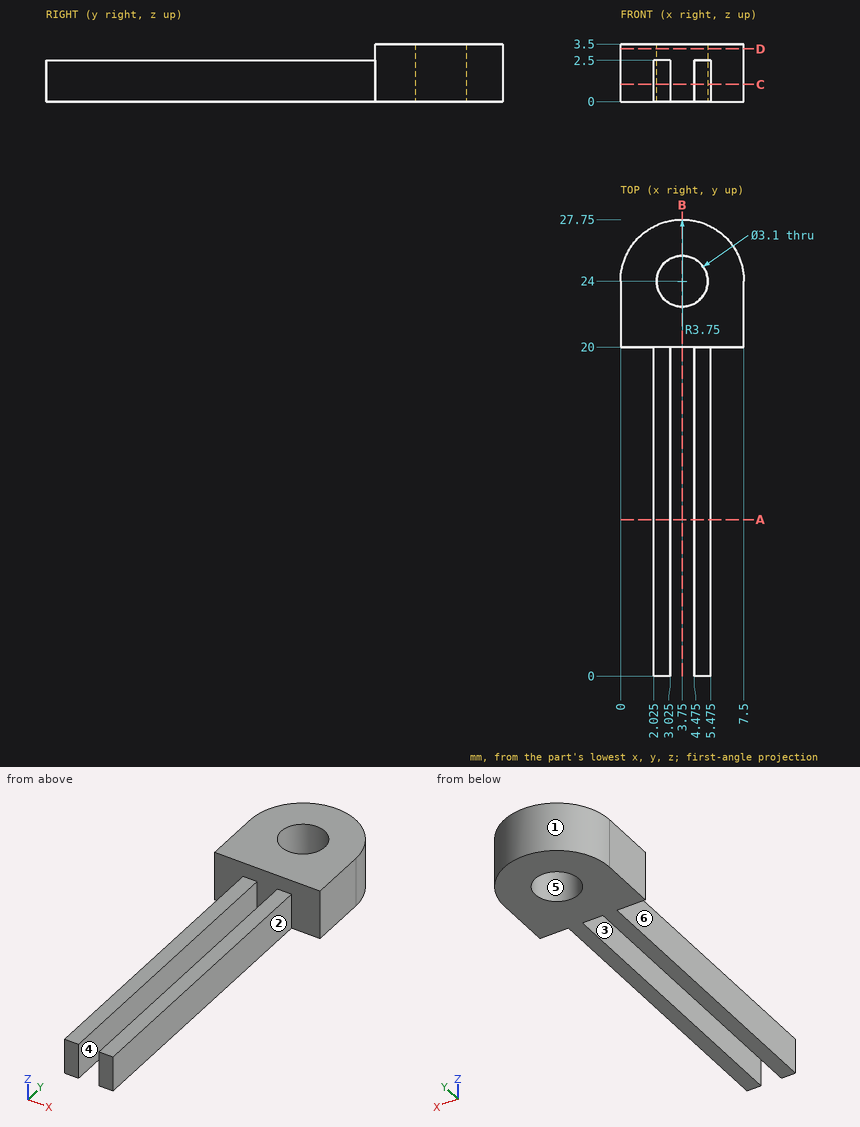
Design review of the part shown in the three views and the two pictorial views. Dimensions are in mm from the part's minimum x, y and z. A direction names the side the tool comes from. Round coordinates to 2 decimals unless told otherwise and drop trailing zeros. Loops run counter-clockwise (first coordinate to the right, second up) from the corner with the lowest first, then second, coordinate; pieces in that order, holes last. Notation, with made-up numbers: (6.25, 17.25) -> (21.25, 17.25) arc R22 ccw to (21.25, 28.25) -> close; hole circle Ø3 at (48.25, 20.5). An arc over 180 degrees is marked (long way). Answer as a JSON object with one key per item and string values. Group by question number.
1) We need section D-D on z = 3.2. Write out the cut boundary in (x, y), then the cut area to 3 significant figures.
2) For the marked faces 4, 5 and 6, list the 3-axis set-ups (+Z, -Z, +X, -X, +Y, -Y) from which the entire face can be reached by the end or side of a thin tool; tool diameter is ignored.
3) We need section C-C on z = 1.05. Write out the cut boundary in (x, y) (3 decimals), then the cut area to 3 significant figures.
4) We need section B-B on x = 3.75. Write out the cut boundary in (y, z).
5) For pin 1 Ø1.1 at (x, y) = (2.5, 8) entering from +Z; pin 2 Ø0.8 at (y, z) = (14.5, 1.5) entering from -X (3 decimals); pin 3 Ø1.9 at (x, y) = (3.75, 24) entering from -Z; pin 4 Ø0.8 at (y, z) = (11.5, 1) entering from +X (3 decimals), all flat-tipped, find the tip position at first contact; note any pin that passes through.
6) Mouldability with a two-part tool opening along X and no side actions: class the marked faces 1, 2 and 3 as released by +X, released by -X, zero draft, split by the parting line, or undercut.
7) We need section A-A on y = 9.5. Write out the cut boundary in (x, z) (3 decimals), then the cut area to 3 significant figures.
8) For line 1 (X direction, y = 19.75, z = 2.45) (3 decimals); line 2 (Y direction, x = 3.75, z = 1.15); line 3 (X direction, y = 24, z = 1.45), list the stretches that pass through material, from the lowest coordinate up. Write a range as [from, to].
Result set:
{
 "1": {"outline": "(0, 20) -> (7.5, 20) -> (7.5, 24) arc R3.75 ccw to (0, 24) -> close; hole circle Ø3.1 at (3.75, 24)", "area": "44.5 mm²"},
 "2": {"face 4": "+Z, -Z, -Y", "face 5": "+Z, -Z", "face 6": "+Z, -Z, -X, -Y"},
 "3": {"outline": "(0, 20) -> (2.025, 20) -> (2.025, 0) -> (3.025, 0) -> (3.025, 20) -> (4.475, 20) -> (4.475, 0) -> (5.475, 0) -> (5.475, 20) -> (7.5, 20) -> (7.5, 24) arc R3.75 ccw to (0, 24) -> close; hole circle Ø3.1 at (3.75, 24)", "area": "84.5 mm²"},
 "4": {"outline": "(20, 0) -> (22.45, 0) -> (22.45, 3.5) -> (20, 3.5) -> close; (25.55, 0) -> (27.75, 0) -> (27.75, 3.5) -> (25.55, 3.5) -> close"},
 "5": {"pin 1": "z = 2.5", "pin 2": "x = 2.025", "pin 3": "through", "pin 4": "x = 5.475"},
 "6": {"face 1": "split by the parting line", "face 2": "released by +X", "face 3": "undercut"},
 "7": {"outline": "(2.025, 0) -> (3.025, 0) -> (3.025, 2.5) -> (2.025, 2.5) -> close; (4.475, 0) -> (5.475, 0) -> (5.475, 2.5) -> (4.475, 2.5) -> close", "area": "5.00 mm²"},
 "8": {"line 1": "[2.025, 3.025], [4.475, 5.475]", "line 2": "[20, 22.45], [25.55, 27.75]", "line 3": "[0, 2.2], [5.3, 7.5]"}
}
